Input: dimensioned drawing with shaded views. Units: mm. Origin: part minimum x, y, z. A direction names the side the tool comes from. Round coordinates to 2 decimals unless told otherwise and drop trailing zeros. Loops run counter-clockwise (first coordinate to the right, second up) from the corner with the lowest first, then second, coordinate; pieces in that order, holes last. Notation, with made-up numbers: M -36,12 L -11,12 A33 ccw -11,44 Z; hole C 33.25,20 d4. An arc over 180 degrees is marked long. Answer as a JSON object with one key per item and string values.
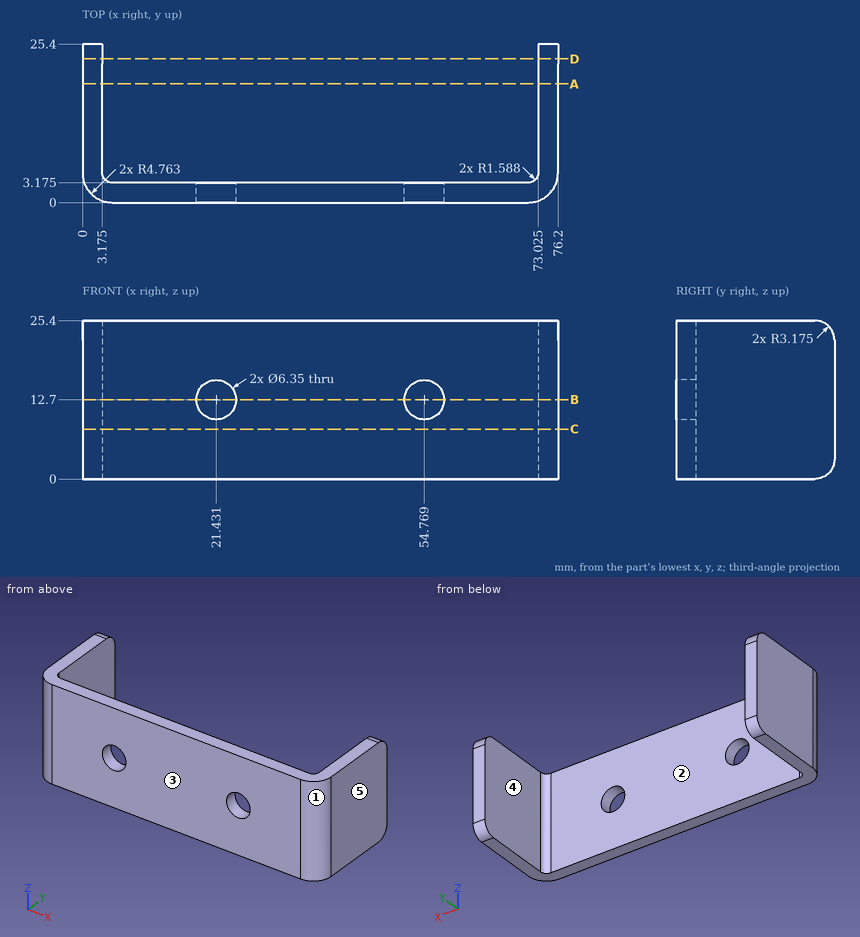
Item 1: Contact query for flat-ended pins moving along their axis: pin 1 Ø1 at (x, z) = (28, 12) entering from +Y (1 decimal); pin 2 Ø7.5 at (x, z) = (54.77, 12.7) entering from -Y. Output: stop coordinate, or through.
Answer sheet:
{"pin 1": "stops at y = 3.2", "pin 2": "stops at y = 0"}
Item 2: Line query: probe 1 along X at (y, z) = (11.5, 14) (1 decimal); probe 2 along X at (y, z) = (1.5, 12.7) (1 decimal); probe 3 along Y at (x, z) = (8, 13.75) (1 decimal). Output: solid intervals per line, ascending. Write a range as from..to.
Answer sheet:
{"probe 1": "x = 0..3.2, 73..76.2", "probe 2": "x = 1.3..18.3, 24.6..51.6, 57.9..74.9", "probe 3": "y = 0..3.2"}
Item 3: Section A-A on y = 19. Return the cut outline in (x, z) (1 decimal).
Answer sheet:
{"outline": "M 0,0 L 3.2,0 L 3.2,25.4 L 0,25.4 Z; M 73,0 L 76.2,0 L 76.2,25.4 L 73,25.4 Z"}
Item 4: Pull-direction query (X, two-part tool) for the marked faces 1, 2 and 3; classes: pulls with the +X half, pulls with the -X half, needs draft (parallel to the pull), parting line crosses it, or undercut.
Answer sheet:
{"face 1": "pulls with the +X half", "face 2": "undercut", "face 3": "needs draft"}
Item 5: Section B-B on z = 12.7. Return the cut outline in (x, y) (1 decimal), then the cut area to 3 significant figures.
Answer sheet:
{"outline": "M 0,4.8 A4.8 ccw 4.8,0 L 18.3,0 L 18.3,3.2 L 4.8,3.2 A1.6 cw 3.2,4.8 L 3.2,25.4 L 0,25.4 Z; M 24.6,0 L 51.6,0 L 51.6,3.2 L 24.6,3.2 Z; M 57.9,0 L 71.4,0 A4.8 ccw 76.2,4.8 L 76.2,25.4 L 73,25.4 L 73,4.8 A1.6 cw 71.4,3.2 L 57.9,3.2 Z", "area": "334 mm²"}
Item 6: Section C-C on z = 8. Return the cut outline in (x, y) (1 decimal).
Answer sheet:
{"outline": "M 0,4.8 A4.8 ccw 4.8,0 L 71.4,0 A4.8 ccw 76.2,4.8 L 76.2,25.4 L 73,25.4 L 73,4.8 A1.6 cw 71.4,3.2 L 4.8,3.2 A1.6 cw 3.2,4.8 L 3.2,25.4 L 0,25.4 Z"}
Item 7: Section D-D on y = 23. Return the cut outline in (x, z) (1 decimal), then the cut area to 3 significant figures.
Answer sheet:
{"outline": "M 0,0.1 L 3.2,0.1 L 3.2,25.3 L 0,25.3 Z; M 73,0.1 L 76.2,0.1 L 76.2,25.3 L 73,25.3 Z", "area": "160 mm²"}
Item 8: Access query for the marked faces 4 and 5. Directions: +Z, -Z, +X, -X, +Y, -Y. A direction counts if a zero-diameter tool reaches every point of the face in a straight line with its end or side. Return the directions, or none.
Answer sheet:
{"face 4": "+Z, -Z, +Y", "face 5": "+Z, -Z, +X, +Y, -Y"}
